Here's how the part is built. I have some questions about the finished solid (model axes, mm). Round coordinates to 2 decimals unless told otherwise and drop trailing zeros. Loops run counter-clockwise (first coordinate to the right, second up) from the corner with the lowest first, then second, coordinate; pieces in that order, holes last. Notation, with made-up numbers: (81.25, 16.25) - (118.25, 16.25) arc R28 ccw to (118.25, 44.25) - close; hole circle Ø7 at (45.25, 63). An arc over 180 degrees is marked (long way). Return JSON: item names as keys, results as strings. Group by question number.
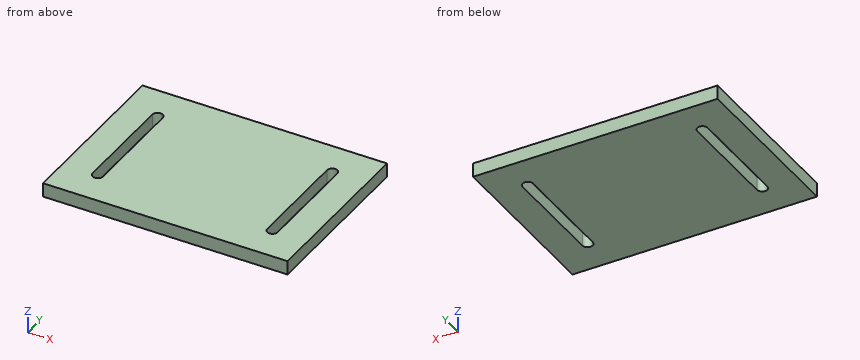
```python
from build123d import *

# Parameters (mm, degrees)
F0_W     = 88.9
F0_H     = 63.5
F1_DEPTH = 5.08
F3_DEPTH = 5.081


with BuildPart() as f1:
    # F0 (on Top) → F1 (new body)
    with BuildSketch(Plane.XY):
        with Locations((44.45, 31.75)):
            Rectangle(F0_W, F0_H)
    extrude(amount=F1_DEPTH)

    # F2 (on face) → F3 (cut, through all)
    with BuildSketch(Plane.XY.offset(5.08)):
        with BuildLine():
            ThreePointArc((14.605, 50.8), (12.7, 52.705), (10.795, 50.8))
            Line((10.795, 50.8), (10.795, 12.7))
            ThreePointArc((10.795, 12.7), (12.7, 10.795), (14.605, 12.7))
            Line((14.605, 12.7), (14.605, 50.8))
        make_face()
        with BuildLine():
            ThreePointArc((78.105, 50.8), (76.2, 52.705), (74.295, 50.8))
            Line((74.295, 50.8), (74.295, 12.7))
            ThreePointArc((74.295, 12.7), (76.2, 10.795), (78.105, 12.7))
            Line((78.105, 12.7), (78.105, 50.8))
        make_face()
    extrude(amount=-F3_DEPTH, mode=Mode.SUBTRACT)


solid = f1.part
```
Q1. Imagine slicing it at B-B, the plane y = 23.5. List the corners of the cut face in (x, z) for me (3 decimals), and give its area (3 significant figures).
Q2. Imagine slicing it at C-C, the plane z = 1.7. List the corners of the cut face in (x, y) for me (3 decimals), and give its area (3 significant figures).
Q3. Please list where this line runs through material, in increasing order: line 1 (X direction, y = 48.5, z = 0.55) (3 decimals).
Q4. Imagine slicing it at A-A, the plane x = 12.7. List the corners of the cut face in (y, z) for me (3 decimals).
Output values:
{
 "1": {"outline": "(0, 0) - (10.795, 0) - (10.795, 5.08) - (0, 5.08) - close; (14.605, 0) - (74.295, 0) - (74.295, 5.08) - (14.605, 5.08) - close; (78.105, 0) - (88.9, 0) - (88.9, 5.08) - (78.105, 5.08) - close", "area": "413 mm^2"},
 "2": {"outline": "(0, 0) - (88.9, 0) - (88.9, 63.5) - (0, 63.5) - close; hole (10.795, 12.7) arc R1.905 ccw to (14.605, 12.7) - (14.605, 50.8) arc R1.905 ccw to (10.795, 50.8) - close; hole (74.295, 12.7) arc R1.905 ccw to (78.105, 12.7) - (78.105, 50.8) arc R1.905 ccw to (74.295, 50.8) - close", "area": "5,330 mm^2"},
 "3": {"line 1": "x = 0 to 10.795, 14.605 to 74.295, 78.105 to 88.9"},
 "4": {"outline": "(0, 0) - (10.795, 0) - (10.795, 5.08) - (0, 5.08) - close; (52.705, 0) - (63.5, 0) - (63.5, 5.08) - (52.705, 5.08) - close"}
}
